from build123d import *

# Parameters (mm, degrees)
SKETCH1_W           = 85
SKETCH1_H           = 67
SKETCH1_R           = 2.1
BOSS_EXTRUDE1_DEPTH = 3
SKETCH1_3_W         = 89
SKETCH1_3_H         = 71
SKETCH1_3_W_2       = 85
SKETCH1_3_H_2       = 67
BOSS_EXTRUDE2_DEPTH = 50
CHAMFER1_SIZE       = 3
SKETCH2_W           = 6
SKETCH2_H           = 6
SKETCH2_R           = 2
BOSS_EXTRUDE3_DEPTH = 32
SKETCH4_W           = 6.06
SKETCH4_H           = 5.26
SKETCH4_R           = 1.625
SKETCH4_W_2         = 5.26
BOSS_EXTRUDE4_DEPTH = 5
SKETCH5_W           = 15
SKETCH5_H           = 20
SKETCH5_W_2         = 17
SKETCH5_H_2         = 11
CUT_EXTRUDE1_DEPTH  = 3
SKETCH7_R           = 4
SKETCH7_W           = 12.5
SKETCH7_H           = 9
CUT_EXTRUDE2_DEPTH  = 10
SKETCH6_W           = 9.543049048
SKETCH6_H           = 11.406034719
SKETCH6_W_2         = 14
SKETCH6_H_2         = 9
SKETCH6_W_3         = 6.1
SKETCH6_H_3         = 6.1
CUT_EXTRUDE3_DEPTH  = 10


with BuildPart() as part:
    # Sketch1 → Boss-Extrude1 (new body)
    with BuildSketch(Plane(origin=(0, 0, 0), x_dir=(1, 0, 0), z_dir=(0, 1, 0))):
        Rectangle(SKETCH1_W, SKETCH1_H)
        with Locations(Location((36.156716418, -28.5, 0), (0, 0, 270))):
            Circle(SKETCH1_R, mode=Mode.SUBTRACT)
        with Locations(Location((36.156716418, 28.5, 0), (0, 0, 270))):
            Circle(SKETCH1_R, mode=Mode.SUBTRACT)
        with Locations(Location((-36.156716418, 28.5, 0), (0, 0, 270))):
            Circle(SKETCH1_R, mode=Mode.SUBTRACT)
    extrude(amount=BOSS_EXTRUDE1_DEPTH)

    # Sketch1<3> → Boss-Extrude2 (add)
    with BuildSketch(Plane(origin=(0, 0, 0), x_dir=(1, 0, 0), z_dir=(0, 1, 0))):
        Rectangle(SKETCH1_3_W, SKETCH1_3_H)
        Rectangle(SKETCH1_3_W_2, SKETCH1_3_H_2, mode=Mode.SUBTRACT)
    extrude(amount=BOSS_EXTRUDE2_DEPTH)

    # Chamfer1
    chamfer1_edges = [part.edges().sort_by_distance(p)[0] for p in [
        (-44.5, 25, -35.5),
        (-44.5, 25, 35.5),
        (44.5, 25, 35.5),
        (44.5, 25, -35.5),
    ]]
    chamfer(chamfer1_edges, length=CHAMFER1_SIZE)

    # Sketch2 → Boss-Extrude3 (add)
    # profile 1 of 3: a face of its own
    with BuildSketch(Plane(origin=(0, 3, 0), x_dir=(1, 0, 0), z_dir=(0, 1, 0))):
        with Locations((-19.5, 30.5)):
            Rectangle(SKETCH2_W, SKETCH2_H)
        with Locations(Location((-19.5, 30.5, 0), (0, 0, 90))):
            Circle(SKETCH2_R, mode=Mode.SUBTRACT)
    # profile 2 of 3: a face of its own
    with BuildSketch(Plane(origin=(0, 3, 0), x_dir=(1, 0, 0), z_dir=(0, 1, 0))):
        with Locations((39.5, 10.5)):
            Rectangle(SKETCH2_W, SKETCH2_H)
        with Locations(Location((39.5, 10.5, 0), (0, 0, 90))):
            Circle(SKETCH2_R, mode=Mode.SUBTRACT)
    # profile 3 of 3: a face of its own
    with BuildSketch(Plane(origin=(0, 3, 0), x_dir=(1, 0, 0), z_dir=(0, 1, 0))):
        with Locations((39.5, -10.5)):
            Rectangle(SKETCH2_W, SKETCH2_H)
        with Locations(Location((39.5, -10.5, 0), (0, 0, 90))):
            Circle(SKETCH2_R, mode=Mode.SUBTRACT)
    extrude(amount=BOSS_EXTRUDE3_DEPTH)

    # Sketch4 → Boss-Extrude4 (add)
    # profile 1 of 4: a face of its own
    with BuildSketch(Plane(origin=(0, 3, 0), x_dir=(1, 0, 0), z_dir=(0, 1, 0))):
        with Locations((-39.47, -30.87)):
            Rectangle(SKETCH4_W, SKETCH4_H)
        with Locations(Location((-39.47, -30.87, 0), (0, 0, 270))):
            Circle(SKETCH4_R, mode=Mode.SUBTRACT)
    # profile 2 of 4: a face of its own
    with BuildSketch(Plane(origin=(0, 3, 0), x_dir=(1, 0, 0), z_dir=(0, 1, 0))):
        with Locations((-23, 22.37)):
            Rectangle(SKETCH4_W_2, SKETCH4_H)
        with Locations(Location((-23, 22.37, 0), (0, 0, 270))):
            Circle(SKETCH4_R, mode=Mode.SUBTRACT)
    # profile 3 of 4: a face of its own
    with BuildSketch(Plane(origin=(0, 3, 0), x_dir=(1, 0, 0), z_dir=(0, 1, 0))):
        with Locations((26.22, 22.37)):
            Rectangle(SKETCH4_W, SKETCH4_H)
        with Locations(Location((26.22, 22.37, 0), (0, 0, 270))):
            Circle(SKETCH4_R, mode=Mode.SUBTRACT)
    # profile 4 of 4: a face of its own
    with BuildSketch(Plane(origin=(0, 3, 0), x_dir=(1, 0, 0), z_dir=(0, 1, 0))):
        with Locations((26.22, -30.87)):
            Rectangle(SKETCH4_W, SKETCH4_H)
        with Locations(Location((26.22, -30.87, 0), (0, 0, 270))):
            Circle(SKETCH4_R, mode=Mode.SUBTRACT)
    extrude(amount=BOSS_EXTRUDE4_DEPTH)

    # Sketch5 → Cut-Extrude1 (cut)
    with BuildSketch(Plane.XY.offset(-33.5)):
        with Locations((15.544213072, 20)):
            Rectangle(SKETCH5_W, SKETCH5_H)
        with Locations((-32.275786928, 5.5)):
            Rectangle(SKETCH5_W_2, SKETCH5_H_2)
    extrude(amount=-CUT_EXTRUDE1_DEPTH, mode=Mode.SUBTRACT)

    # Sketch7 → Cut-Extrude2 (cut)
    with BuildSketch(Plane(origin=(44.5, 0, 0), x_dir=(0, 0, -1), z_dir=(1, 0, 0))):
        with Locations((-23, 19)):
            Circle(SKETCH7_R)
        with Locations((2, 24.5)):
            Rectangle(SKETCH7_W, SKETCH7_H)
    extrude(amount=-CUT_EXTRUDE2_DEPTH, mode=Mode.SUBTRACT)

    # Sketch6 → Cut-Extrude3 (cut)
    with BuildSketch(Plane(origin=(-42.5, 0, 0), x_dir=(0, 0, -1), z_dir=(1, 0, 0))):
        with Locations((17.512756781, 15.365129708)):
            Rectangle(SKETCH6_W, SKETCH6_H)
        with Locations((-17.5, 38.5)):
            Rectangle(SKETCH6_W_2, SKETCH6_H_2)
        with Locations((21.45, 39.95)):
            Rectangle(SKETCH6_W_3, SKETCH6_H_3)
    extrude(amount=-CUT_EXTRUDE3_DEPTH, mode=Mode.SUBTRACT)


solid = part.part
For this review, take the finished solid that the model builds, in its own axes (mm). A direction names the side the tool comes from. Round coordinates to 2 decimals unless told otherwise and drop trailing zeros. Loops run counter-clockwise (first coordinate to the right, second up) from the corner with the lowest first, then second, coordinate; pieces in that order, holes last. Notation, with made-up numbers: (76.5, -14.75) - (111.5, -14.75) arc R20 ccw to (111.5, 10.25) - close; hole circle Ø8 at (55.5, -25). An arc over 180 degrees is marked (long way). Use one line per item in the form item = value.
1) Mouldability with a two-part tool opening along X and no side actions: class faces 1 (the face through (26.2, 8, -24.2)), 2 (the face through (-43, 15, -12.741)), 3 (the face through (-1, 26, 33.5)) as pulls with the +X half, pulls with the -X half, needs draft (parallel to the pull), parting line crosses it, or undercut.
Solutions:
face_1 = undercut
face_2 = needs draft
face_3 = undercut
2) Clearance check with flat-ended pins moving along their axes: P1, Ø1.5, axis at x = -29, z = 21.5, coming from the +Y side; P2, Ø2, axis at x = 40, z = 9.5, coming from the +Y side; P3, Ø0.6, axis at y = 4, z = -34.5, coming from the -X side; P4, Ø2, axis at x = -43.5, z = -21.5, coming from the -Y side. State where each tip first meets the part, or that it passes through.
Solutions:
P1 = 3
P2 = 35
P3 = -42.8
P4 = 0
3) Tool access review of faces 4 (the face through (0, 50, 34)), 5 (the face through (-43, 36.9, -21)), 6 (the face through (-42.5, 26, 0)), 7 (the face through (-36.44, 5, 31)), 8 (the face through (15, 30, -34)): name each direction out of +Z, -Z, +X, -X, +Y, -Y from which nothing blocks a thin tool from reaching the whole face with its end or side.
Solutions:
face_4 = +Z, -Z, +X, -X, +Y
face_5 = -X
face_6 = +Y
face_7 = -Z, +Y
face_8 = -Z
4) We need section B-B on y = 38. Write out the cut boundary in (x, z), then the cut area to 3 significant figures.
Solutions:
outline = (-44.5, -32.5) - (-41.5, -35.5) - (41.5, -35.5) - (44.5, -32.5) - (44.5, 32.5) - (41.5, 35.5) - (-41.5, 35.5) - (-44.5, 32.5) - (-44.5, 24.5) - (-42.5, 24.5) - (-42.5, 33.5) - (42.5, 33.5) - (42.5, -33.5) - (-42.5, -33.5) - (-42.5, -24.5) - (-44.5, -24.5) - close; (-44.5, -18.4) - (-42.5, -18.4) - (-42.5, 10.5) - (-44.5, 10.5) - close
area = 566 mm2
5) We need section A-A on x = -39.47. Write out the cut boundary in (y, z) (3 decimals), then the cut area to 3 significant figures.
Solutions:
outline = (0, -33.5) - (3, -33.5) - (3, 28.24) - (8, 28.24) - (8, 29.245) - (3, 29.245) - (3, 32.495) - (8, 32.495) - (8, 33.5) - (50, 33.5) - (50, 35.5) - (0, 35.5) - close; (11, -35.5) - (50, -35.5) - (50, -33.5) - (11, -33.5) - close
area = 389 mm2
6) Wall thickness on probe 1 along Z at (x, y) = (39.5, 11); probe 2 along Z at (x, y) = (-19.5, 16); probe 3 along X at (y, z) = (25.5, -10.5): over which ranges is each line inside the solid? List them lowest first.
Solutions:
probe_1 = -35.5 to -33.5, -13.5 to -12.5, -8.5 to -7.5, 7.5 to 8.5, 12.5 to 13.5, 33.5 to 35.5
probe_2 = -35.5 to -32.5, -28.5 to -27.5, 33.5 to 35.5
probe_3 = -44.5 to -42.5, 36.5 to 37.5, 41.5 to 44.5
7) We need section C-C on z = 17. Write out the cut boundary in (x, y).
Solutions:
outline = (-44.5, 0) - (44.5, 0) - (44.5, 50) - (42.5, 50) - (42.5, 3) - (-42.5, 3) - (-42.5, 34) - (-44.5, 34) - close; (-44.5, 43) - (-42.5, 43) - (-42.5, 50) - (-44.5, 50) - close
8) We need section D-D on y = 19. State how many separate pieces and enclosed holes the cut face has, then the cut area to 3 significant figures.
Solutions:
separate_pieces = 3
enclosed_holes = 3
area = 611 mm2
